Input: dimensioned drawing with shaded views. Units: mm. Origin: part minimum x, y, z. Round coordinates to 2 decimals unless told otherwise and drop trailing zeros. Write each loop counter-clockwise with the first axis right and the second up, starting at its lowest first coordinate (ties: lowest second). Pieces come first, ordered by that corner, then holes. Notation, with made-up numbers: (-13, -27.75) -> (44, -27.75) arc R18 cw to (44, -11.75) -> close; hole circle Ø7 at (39, 14). An arc over 180 degrees is marked (long way). One line per item, written item: value. Start each with the question number.
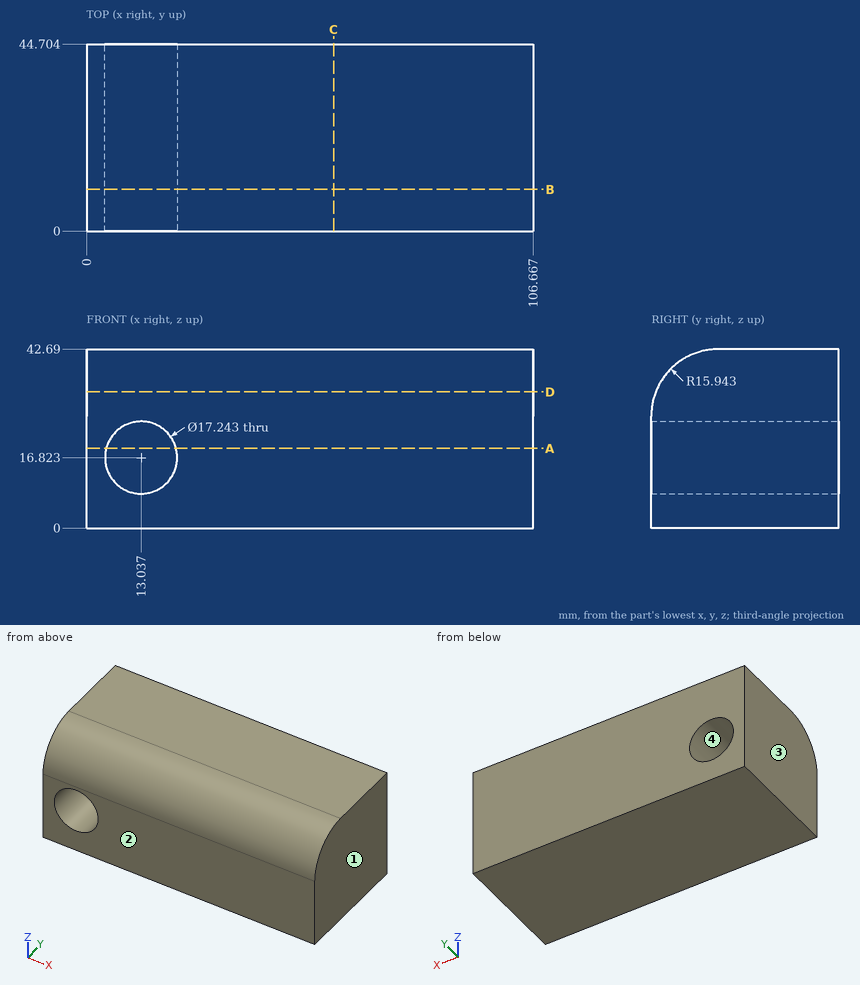
(1) Line query: probe 1 along X at (y, z) = (4, 16.5); probe 2 along X at (y, z) = (35.5, 10.5) (1 decimal); probe 3 along Z at (x, y) = (15, 20). Output: solid intervals per line, ascending.
(2) Pull-direction query (X, two-part tool) for the marked faces 1, 2, 3 and 4; classes: pulls with the +X half, pulls with the -X half, needs draft (parallel to the pull), parting line crosses it, or undercut.
(3) Section query B-B (y = 10). Output: boundary loops of the cut face in (x, z), and give its area (3 significant figures).
(4) Pin query (flat end, axial travel): pin 1 (4 mm diameter, centred on x = 46.5, y = 11, fed in from +Z) (1 decimal); pin 2 (15.5 mm diameter, centred on x = 13.04, z = 16.82, fed in from +Y); pin 3 (8 mm diameter, centred on x = 62.5, y = 10.5, fed in from +Z); pin 4 (4 mm diameter, centred on x = 59, z = 31.5, fed in from -Y). Return the tip coordinate at first contact, or that it passes through.
(5) Section query D-D (z = 32.5). Output: boundary loops of the cut face in (x, y) (1 decimal), and give its area (3 significant figures).
(6) Section query A-A (z = 19). Output: boundary loops of the cut face in (x, y) (1 decimal), and give its area (3 significant figures).
(7) Section query C-C (x = 59). Output: boundary loops of the cut face in (y, z), and give its area (3 significant figures).
Results list:
1. probe 1: x = 0 to 4.42, 21.65 to 106.67
1. probe 2: x = 0 to 7.2, 18.9 to 106.7
1. probe 3: z = 0 to 8.43, 25.22 to 42.69
2. face 1: pulls with the +X half
2. face 2: needs draft
2. face 3: pulls with the -X half
2. face 4: undercut
3. outline: (0, 0) -> (106.67, 0) -> (106.67, 41.54) -> (0, 41.54) -> close; hole circle Ø17.24 at (13.04, 16.82)
3. area: 4,200 mm^2
4. pin 1: stops at z = 42.4
4. pin 2: passes through
4. pin 3: stops at z = 42.62
4. pin 4: stops at y = 0.24
5. outline: (0, 1.1) -> (106.7, 1.1) -> (106.7, 44.7) -> (0, 44.7) -> close
5. area: 4,650 mm^2
6. outline: (0, 0) -> (4.7, 0) -> (4.7, 44.7) -> (0, 44.7) -> close; (21.4, 0) -> (106.7, 0) -> (106.7, 44.7) -> (21.4, 44.7) -> close
6. area: 4,020 mm^2
7. outline: (0, 0) -> (44.7, 0) -> (44.7, 42.69) -> (15.94, 42.69) arc R15.94 ccw to (0, 26.75) -> close
7. area: 1,850 mm^2
